Answer from the drawing. Dimensions are ordinates in mm from the lowest x, y and z of the part. Round coordinates to 2 decimals unless told otherwise and drop trailing zeros. Loops run counter-clockwise (first coordinate to the right, second up) from the corner with the lowest first, then second, coordinate; pieces in that order, holes last. Notation, with made-up numbers: (-9, -16.5) - (3, -16.5) arc R8 ccw to (3, -12.5) - close; hole circle Ø6 at (23.25, 77.25). An arc over 180 degrees is marked (long way). Return JSON: item names as keys, results as strings.
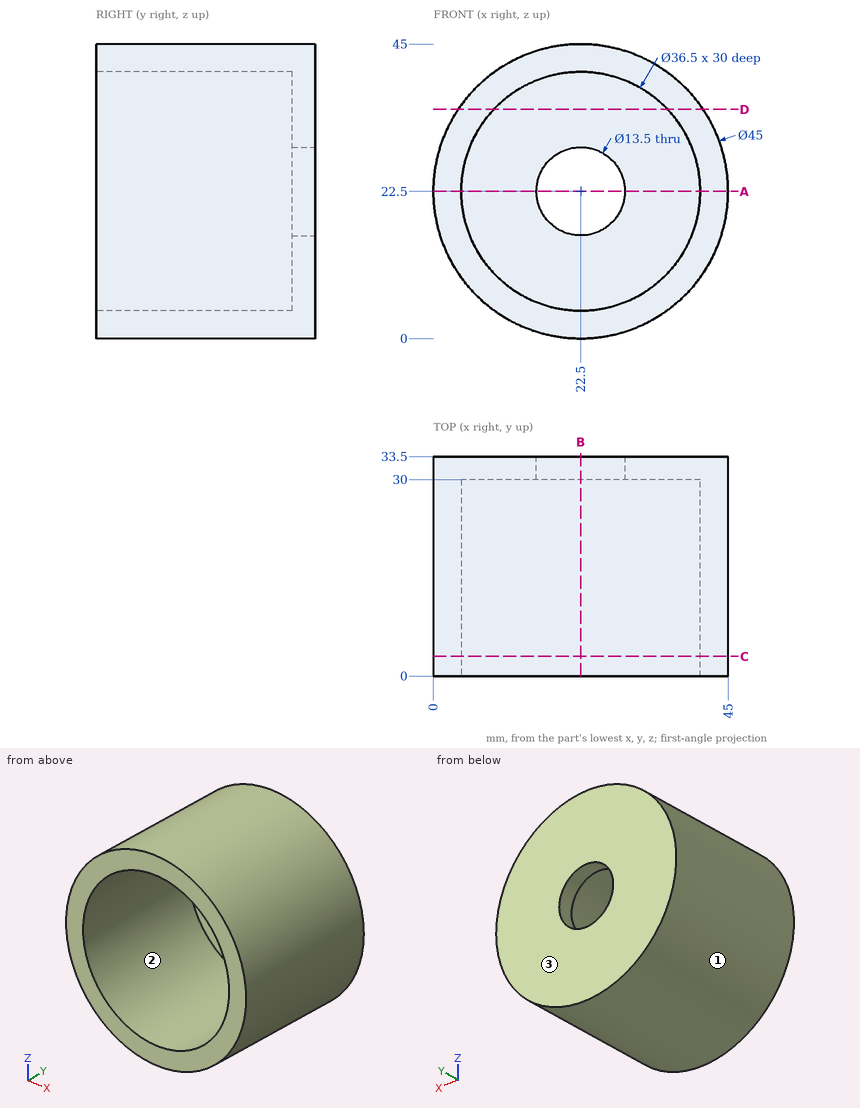
1) Section D-D (z = 35) is taken. Give the vertices of the cut face in (x, y), and give its area (3 significant figures).
Verdict:
{"outline": "(3.79, 0) - (9.2, 0) - (9.2, 30) - (35.8, 30) - (35.8, 0) - (41.21, 0) - (41.21, 33.5) - (3.79, 33.5) - close", "area": "456 mm2"}
2) Flat-ended cylindrical pins translate along their axes: pin 1 (8 mm diameter, centred on x = 27.5, y = 7.5, fed in from +Z); pin 2 (4 mm diameter, centred on y = 4, z = 29, fed in from +X); pin 3 (12 mm diameter, centred on x = 39, z = 38.5, fed in from -Y); pin 4 (6 mm diameter, centred on x = 28, z = 21, fed in from -Y). Find the tip coordinate at first contact, or state that the pin passes through.
Verdict:
{"pin 1": "stops at z = 44.98", "pin 2": "stops at x = 44.55", "pin 3": "stops at y = 0", "pin 4": "stops at y = 30"}
3) Determine the mould class of the marked faces 1, 2 and 3 for opening direction Z: pulls with the +Z half, pulls with the -Z half, needs draft (parallel to the pull), parting line crosses it, or undercut.
Verdict:
{"face 1": "parting line crosses it", "face 2": "undercut", "face 3": "needs draft"}
4) Section C-C (y = 3) is taken. Give the vertices of the cut face in (x, z), and give its area (3 significant figures).
Verdict:
{"outline": "circle Ø45 at (22.5, 22.5); hole circle Ø36.5 at (22.5, 22.5)", "area": "544 mm2"}
5) Section A-A (z = 22.5) is taken. Give the vertices of the cut face in (x, y).
Verdict:
{"outline": "(0, 0) - (4.25, 0) - (4.25, 30) - (15.75, 30) - (15.75, 33.5) - (0, 33.5) - close; (29.25, 30) - (40.75, 30) - (40.75, 0) - (45, 0) - (45, 33.5) - (29.25, 33.5) - close"}
6) Section B-B (x = 22.5) is taken. Give the vertices of the cut face in (y, z).
Verdict:
{"outline": "(0, 0) - (33.5, 0) - (33.5, 15.75) - (30, 15.75) - (30, 4.25) - (0, 4.25) - close; (0, 40.75) - (30, 40.75) - (30, 29.25) - (33.5, 29.25) - (33.5, 45) - (0, 45) - close"}
7) Find the intervals of material crossed by L1, parallel to X at y = 32.1, z = 22.5; L2, parallel to Z at x = 22, y = 15, in increasing order.
Verdict:
{"L1": "x = 0 to 15.75, 29.25 to 45", "L2": "z = 0.01 to 4.26, 40.74 to 44.99"}
